Could you check a few things on this model? Use its own coordinates, in mm. A direction names the side the tool comes from. Round coordinates to 2 decimals unless told otherwise and drop trailing zeros. Loops run counter-clockwise (first coordinate to the right, second up) from the corner with the lowest first, then second, coordinate; pieces in that order, holes last. Notation, with made-up numbers: (18, 87.5) -> (35, 87.5) arc R11 ccw to (35, 102.5) -> close; hole circle Ø2 at (12.25, -22). An arc over 180 degrees is marked (long way). One line per item, written item: value.
from build123d import *

# Parameters (mm, degrees)
F0_W     = 15
F0_H     = 15
F1_DEPTH = 15
F2_R     = 2
F3_R     = 3
F4_DEPTH = 2


with BuildPart() as f1:
    # F0 (on Front) → F1 (new body)
    with BuildSketch(Plane.XZ):
        Rectangle(F0_W, F0_H)
    extrude(amount=-F1_DEPTH)

    # F2
    f2_edges = [f1.edges().sort_by_distance(p)[0] for p in [
        (7.5, 7.5, 7.5),
        (-7.5, 7.5, 7.5),
        (0, 0, 7.5),
        (0, 15, 7.5),
        (7.5, 7.5, -7.5),
        (7.5, 0, 0),
        (7.5, 15, 0),
        (-7.5, 0, 0),
        (0, 0, -7.5),
        (-7.5, 7.5, -7.5),
        (0, 15, -7.5),
        (-7.5, 15, 0),
    ]]
    fillet(f2_edges, radius=F2_R)

    # F3 (on face) → F4 (cut)
    with BuildSketch(Plane.XZ):
        Circle(F3_R)
    extrude(amount=-F4_DEPTH, mode=Mode.SUBTRACT)


solid = f1.part
(1) I'm going to push a flat-ended pin straight in: pin 1 Ø1.8 at (x, z) = (1, 1.5) entering from -Y. Where does the tip first touch, or does it pass through?
Recorded:
pin 1: y = 2
(2) If we section it at A-A, the plane x = 0: Please give me the cut outline in (y, z).
Recorded:
outline: (0, -5.5) arc R2 ccw to (2, -7.5) -> (13, -7.5) arc R2 ccw to (15, -5.5) -> (15, 5.5) arc R2 ccw to (13, 7.5) -> (2, 7.5) arc R2 ccw to (0, 5.5) -> (0, 3) -> (2, 3) -> (2, -3) -> (0, -3) -> close
(3) If we section it at B-B, the plane z = 0: Please give me the cut outline in (x, y).
Recorded:
outline: (-7.5, 2) arc R2 ccw to (-5.5, 0) -> (-3, 0) -> (-3, 2) -> (3, 2) -> (3, 0) -> (5.5, 0) arc R2 ccw to (7.5, 2) -> (7.5, 13) arc R2 ccw to (5.5, 15) -> (-5.5, 15) arc R2 ccw to (-7.5, 13) -> close
(4) If I drill on L1, parallel to Y at x = -1.5, z = 2.5; L2, parallel to Z at x = 0, y = 1.45; L3, parallel to Z at x = 0, y = 0.65, over which ranges is the centre line in solid material (lowest first)?
Recorded:
L1: 2 to 15
L2: -7.42 to -3, 3 to 7.42
L3: -6.98 to -3, 3 to 6.98
(5) If we section it at D-D, the plane y = 1.75: Please give me the cut outline in (x, z), then the cut area to 3 significant figures.
Recorded:
outline: (-7.48, -5.5) arc R1.98 ccw to (-5.5, -7.48) -> (5.5, -7.48) arc R1.98 ccw to (7.48, -5.5) -> (7.48, 5.5) arc R1.98 ccw to (5.5, 7.48) -> (-5.5, 7.48) arc R1.98 ccw to (-7.48, 5.5) -> close; hole circle Ø6 at (0, 0)
area: 192 mm²
(6) For faces 5 (the face through (0.08, 0.6, -6.93)), 6 (the face through (-3, 1, 0)), which set-ups out of +Z, -Z, +X, -X, +Y, -Y let a thin tool reach every point of the face, with its end or its side?
Recorded:
face 5: -Z, +X, -X, -Y
face 6: -Y
(7) If we section it at C-C, the plane y = 12.75: Please give me the cut outline in (x, z), then the cut area to 3 significant figures.
Recorded:
outline: (-7.5, -5.5) arc R2 ccw to (-5.5, -7.5) -> (5.5, -7.5) arc R2 ccw to (7.5, -5.5) -> (7.5, 5.5) arc R2 ccw to (5.5, 7.5) -> (-5.5, 7.5) arc R2 ccw to (-7.5, 5.5) -> close
area: 222 mm²
(8) Thinking about a two-plate mould opening in Z: for faces 1 (the face through (-6.93, 7.58, -6.9)), 2 (the face through (0, 15, 0)), 3 (the face through (0, 7, 7.5)), 4 (the face through (0, 2, 0)), which applies, released by +Z, released by -Z, zero draft, split by the parting line, or undercut?
Recorded:
face 1: released by -Z
face 2: zero draft
face 3: released by +Z
face 4: undercut
